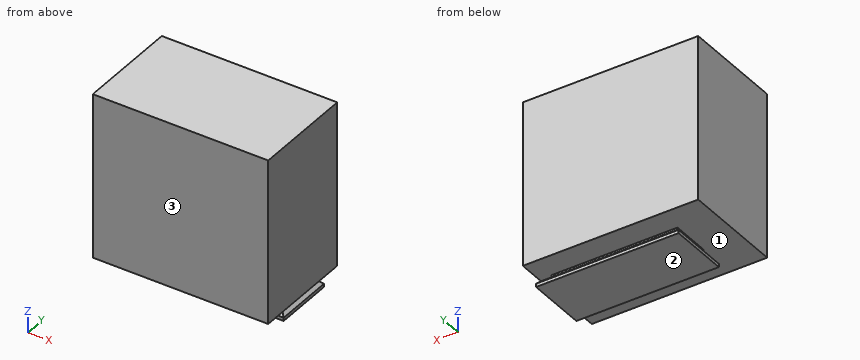
Autodesk Inventor part; units mm, degrees
ref_plane "YZ Plane" through (0, 0, 0) normal (1, 0, 0) x (0, 1, 0)
ref_plane "XZ Plane" through (0, 0, 0) normal (0, 1, 0) x (-1, 0, 0)
ref_plane "XY Plane" through (0, 0, 0) normal (0, 0, 1) x (1, 0, 0)
sketch "Sketch1" plane through (0, 0, 0) normal (0, 0, 1) x (1, 0, 0)
  line L0 (-21.65, 9.15) -> (21.65, 9.15)
  line L1 (21.65, 9.15) -> (21.65, -9.15)
  line L2 (21.65, -9.15) -> (-21.65, -9.15)
  line L3 (-21.65, -9.15) -> (-21.65, 9.15)
  line L4 (-21.65, 9.15) -> (21.65, -9.15) construction
  line L5 (21.65, 9.15) -> (-21.65, -9.15) construction
  point P0 (0, 0)
  dimension "d0" = 43.3
  dimension "d1" = 18.3
extrude "Extrusion1" add sketch "Sketch1" along normal blind 2
sketch "Sketch2" plane through (0, 0, 2) normal (0, 0, 1) x (1, 0, 0)
  line L0 (-19.15, 5.9) -> (19.15, 5.9)
  line L1 (19.15, 5.9) -> (19.15, -5.9)
  line L2 (19.15, -5.9) -> (-19.15, -5.9)
  line L3 (-19.15, -5.9) -> (-19.15, 5.9)
  line L4 (-19.15, 5.9) -> (19.15, -5.9) construction
  line L5 (19.15, 5.9) -> (-19.15, -5.9) construction
  point P0 (0, 0)
  dimension "d4" = 38.3
  dimension "d5" = 11.8
extrude "Extrusion2" add sketch "Sketch2" along normal blind 2.5
chamfer "Chamfer1" distance 1 angle 45 4 edges at (0, -9.15, 2) (21.65, 0, 2) (-21.65, 0, 2) (0, 9.15, 2)
sketch "Sketch3" plane through (0, 0, 4.5) normal (0, 0, 1) x (1, 0, 0)
  line L0 (22.8185, -17.9) -> (-30.4815, -17.9)
  line L1 (-30.4815, -17.9) -> (-30.4815, 13.4)
  line L2 (-30.4815, 13.4) -> (22.8185, 13.4)
  line L3 (22.8185, 13.4) -> (22.8185, -17.9)
  line L4 (-30.4815, -17.9) -> (22.8185, 13.4) construction
  line L5 (19.15, 5.9) -> (-19.15, 5.9)
  line L6 (-19.15, -5.9) -> (19.15, -5.9)
  point P0 (0, 0)
  dimension "d11" = 53.3
  dimension "d12" = 7.5
  dimension "d13" = 12
extrude "Extrusion3" add sketch "Sketch3" along normal blind 50
properties part number "Power Socket Insert v1"
Design review of the part built by this model. Coordinates are the model's own, in mm. Face numbers are marked on the shaded views. Round coordinates to 2 decimals unless told otherwise and drop trailing zeros. Write each loop counter-clockwise with the first axis right and the second up, starting at its lowest first coordinate (ties: lowest second). Pieces come first, ordered by that corner, then holes. Notation, with made-up numbers: (77.25, 51) -> (99.25, 51) arc R32 cw to (99.25, 79) -> close; hole circle Ø5 at (-4, 23). An arc over 180 degrees is marked (long way). One line per item, written item: value. Start each with the question number.
Q1. To check wall thickness, follow probe 1 along Z at (x, y) = (-20, -7.5); probe 2 along Z at (x, y) = (-25.5, -14); probe 3 along Z at (x, y) = (15.5, -9). State the ranges of each line that lie inside material, in increasing order.
Q2. Add section C-C (x = -25.5). Give the boundary of the cut face in (y, z).
Q3. The part is to be moulded in two halves that separate along Z. For the marked faces 1, 2 and 3, say which applies: pulls with the +Z half, pulls with the -Z half, needs draft (parallel to the pull), parting line crosses it, or undercut.
Q4. Add section A-A (y = -3.5). Give the boundary of the cut face in (x, z), then the cut area to 3 significant figures.
Q5. Add section B-B (x = -11). Give the boundary of the cut face in (y, z).
Q6. Insertion check: P1, Ø0.8, axis at y = 2.5, z = 0.5, coming from the -X side; P2, Ø0.5, axis at y = -1, z = 0.5, coming from the +X side; P3, Ø1.2, axis at y = -1.5, z = 3, coming from the -X side. Each pin has a flat end and moves straight along its axis. Give the tip position at first contact, or say it passes through.
Response:
1. probe 1: z = 0 to 2, 4.5 to 54.5
1. probe 2: z = 4.5 to 54.5
1. probe 3: z = 0 to 1.15, 4.5 to 54.5
2. outline: (-17.9, 4.5) -> (13.4, 4.5) -> (13.4, 54.5) -> (-17.9, 54.5) -> close
3. face 1: undercut
3. face 2: pulls with the -Z half
3. face 3: needs draft
4. outline: (-30.48, 4.5) -> (-19.15, 4.5) -> (-19.15, 2) -> (-20.65, 2) -> (-21.65, 1) -> (-21.65, 0) -> (21.65, 0) -> (21.65, 1) -> (20.65, 2) -> (19.15, 2) -> (19.15, 4.5) -> (22.82, 4.5) -> (22.82, 54.5) -> (-30.48, 54.5) -> close
4. area: 2,850 mm^2
5. outline: (-17.9, 4.5) -> (-5.9, 4.5) -> (-5.9, 2) -> (-8.15, 2) -> (-9.15, 1) -> (-9.15, 0) -> (9.15, 0) -> (9.15, 1) -> (8.15, 2) -> (5.9, 2) -> (5.9, 4.5) -> (13.4, 4.5) -> (13.4, 54.5) -> (-17.9, 54.5) -> close
6. P1: stops at x = -21.65
6. P2: stops at x = 21.65
6. P3: stops at x = -19.15
